Source: CAD feature listing. Evaluate the final solid. Frame: model axes, mm. A direction names the side the tool comes from. Round coordinates to 2 decimals unless told otherwise and drop trailing zeros. Loops run counter-clockwise (first coordinate to the right, second up) from the corner with the lowest first, then second, coordinate; pieces in that order, holes last. Notation, with made-up numbers: (54, 14.5) -> (89, 14.5) arc R22 cw to (89, 34.5) -> close; hole circle Ø6 at (81.5, 36). An arc over 180 degrees is marked (long way). Write item = value, one per line.
from build123d import *

# Parameters (mm, degrees)
F0_R     = 175
F1_DEPTH = 25
F2_R     = 15
F3_DEPTH = 600
F4_R     = 55
F4_R_2   = 15
F5_DEPTH = 5
F6_R     = 50
F7_DEPTH = 10
F8_R     = 55
F8_R_2   = 50
F9_DEPTH = 5


with BuildPart() as f1:
    # F0 (on Top) → F1 (new body)
    with BuildSketch(Plane.XY):
        Circle(F0_R)
    extrude(amount=F1_DEPTH)

    # F2 (on face) → F3 (join)
    with BuildSketch(Plane(origin=(0, 0, 0), x_dir=(1, 0, 0), z_dir=(0, 0, -1))):
        Circle(F2_R)
    extrude(amount=F3_DEPTH)

    # F4 (on face) → F5 (join)
    with BuildSketch(Plane(origin=(0, 0, -600), x_dir=(1, 0, 0), z_dir=(0, 0, -1))):
        Circle(F4_R)
        Circle(F4_R_2, mode=Mode.SUBTRACT)
        Circle(F4_R_2)
    extrude(amount=F5_DEPTH)

    # F6 (on face) → F7 (join)
    with BuildSketch(Plane(origin=(0, 0, -605), x_dir=(1, 0, 0), z_dir=(0, 0, -1))):
        Circle(F6_R)
    extrude(amount=F7_DEPTH)

    # F8 (on face) → F9 (join)
    with BuildSketch(Plane(origin=(0, 0, -615), x_dir=(1, 0, 0), z_dir=(0, 0, -1))):
        Circle(F8_R)
        Circle(F8_R_2, mode=Mode.SUBTRACT)
        Circle(F8_R_2)
    extrude(amount=F9_DEPTH)


solid = f1.part
1. Set-up query: faces 4 (the face through (12, 49, -615)), 5 (the face through (-11.923, 53.692, -602.465)), 6 (the face through (-1, -1, -620)). Return all of +Z, -Z, +X, -X, +Y, -Y with unobstructed straight access to the full face (end or side cutting, diameter ignored); none if empty.
Evaluation:
face_4 = none
face_5 = -Z
face_6 = -Z, +X, -X, +Y, -Y
2. Mould query, pull axis Z, two halves, no side actions, for faces 1 (the face through (-14.985, -0.66, -295.8)), 2 (the face through (-128.982, 118.273, 12.325)), 3 (the face through (-2, 2, 25)). Classes: released by +Z, released by -Z, zero draft, split by the parting line, or undercut.
Evaluation:
face_1 = undercut
face_2 = zero draft
face_3 = released by +Z
3. Section query C-C (z = -220). Return the cut outline in (x, y).
Evaluation:
outline = circle Ø30 at (0, 0)
4. Section query B-B (x = 0). Return the cut outline in (y, z).
Evaluation:
outline = (-175, 0) -> (-15, 0) -> (-15, -600) -> (-55, -600) -> (-55, -605) -> (-50, -605) -> (-50, -615) -> (-55, -615) -> (-55, -620) -> (55, -620) -> (55, -615) -> (50, -615) -> (50, -605) -> (55, -605) -> (55, -600) -> (15, -600) -> (15, 0) -> (175, 0) -> (175, 25) -> (-175, 25) -> close
5. Contact query for flat-ended pins moving along their axis: pin 1 Ø1.5 at (y, z) = (6, -139) entering from -X; pin 2 Ø6 at (x, z) = (-6, -366) entering from +Y. Output: stop coordinate, or through.
Evaluation:
pin_1 = -14.05
pin_2 = 14.7
6. Section query D-D (y = 77). Return the cut outline in (x, z).
Evaluation:
outline = (-157.15, 0) -> (157.15, 0) -> (157.15, 25) -> (-157.15, 25) -> close
7. Line query: probe 1 along Z at (x, y) = (49.5, 14.5); probe 2 along Z at (x, y) = (-34, -34); probe 3 along Z at (x, y) = (73.5, 28). Output: solid intervals per line, ascending. Write a range as from..to.
Evaluation:
probe_1 = -620..-615, -605..-600, 0..25
probe_2 = -620..-600, 0..25
probe_3 = 0..25
8. Section query A-A (y = 26). Return the cut outline in (x, z), then the cut area to 3 significant figures.
Evaluation:
outline = (-173.06, 0) -> (173.06, 0) -> (173.06, 25) -> (-173.06, 25) -> close; (-48.47, -620) -> (48.47, -620) -> (48.47, -615) -> (42.71, -615) -> (42.71, -605) -> (48.47, -605) -> (48.47, -600) -> (-48.47, -600) -> (-48.47, -605) -> (-42.71, -605) -> (-42.71, -615) -> (-48.47, -615) -> close
area = 10,500 mm²
